For this review, take the finished solid that the model builds, in its own axes (mm). Face numbers are marked on the shaded views. A direction names the side the tool comes from. Round coordinates to 2 decimals unless told otherwise and drop trailing zeros. Loops run counter-clockwise (first coordinate to the right, second up) from the corner with the lowest first, then second, coordinate; pieces in that order, holes last. Notation, with made-up numbers: M -9.5,14 L 31.5,14 A9 ccw 31.5,31 Z; hole C -31,-38.75 d3. An arc over 180 degrees is marked long. Write item = value, one per line. Start each with the question number.
```python
from build123d import *

# Parameters (mm, degrees)
F0_W     = 95.25
F0_H     = 31.75
F1_DEPTH = 88.9
F2_T     = -2.54
F4_D     = 7.9375
F4_DEPTH = 12.7
F5_W     = 15.24
F5_H     = 12.065
F6_DEPTH = 2.54


with BuildPart() as f1:
    # F0 (on Front) → F1 (new body)
    with BuildSketch(Plane.XZ):
        Rectangle(F0_W, F0_H)
    extrude(amount=F1_DEPTH)

    # F2
    f2_openings = [f1.faces().sort_by_distance(p)[0] for p in [
        (0, -44.45, 15.875),
    ]]
    offset(amount=F2_T, openings=f2_openings)

    # F4
    with Locations(Plane.XZ.offset(88.9)):
        with Locations((23.771884, 0)):
            Hole(F4_D / 2, depth=F4_DEPTH)

    # F5 (on face) → F6 (cut, through all)
    with BuildSketch(Plane.XZ.offset(88.9)):
        with Locations((-24.736177, 2.730849)):
            Rectangle(F5_W, F5_H)
    extrude(amount=-F6_DEPTH, mode=Mode.SUBTRACT)


solid = f1.part
```
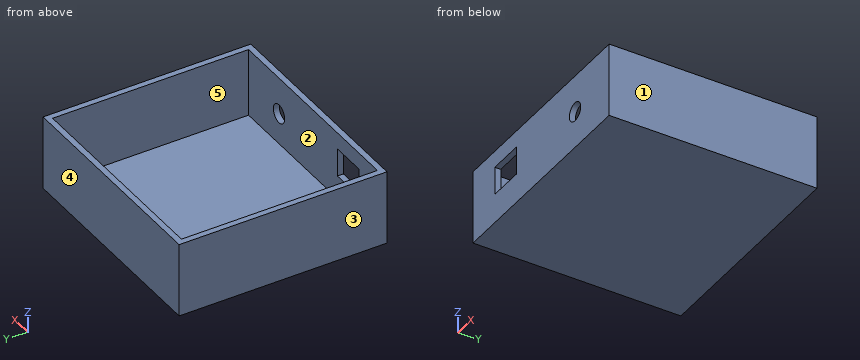
(1) Wall thickness on L1, parallel to Y at x = 10, z = 1; L2, parallel to X at y = -10.5, z = 9 (3 decimals); L3, parallel to Z at x = 19, y = -56 (3 decimals): over which ranges is each line inside the solid? List them lowest first.
(2) For pin 1 Ø5 at (x, z) = (23.77, 0) entering from -Y; pin 2 Ø8 at (x, y) = (-24, -23) entering from +Z (3 decimals), all flat-tipped, find the tip position at first contact; note any pin that passes through.
(3) Add section B-B on x = 21. Write out the cut boundary in (y, z) (3 decimals).
(4) Draft analysis for pull direction X (two halves, no side actions). For the marked faces 3, 4 and 5, state which applies: +X half, -X half, draft (parallel to the pull), parting line (faces both ways), or undercut.
(5) Add section A-A on z = 0. Write out the cut boundary in (x, y) (3 decimals).
(6) Tool access review of the marked faces 1 and 2: name each direction out of +Z, -Z, +X, -X, +Y, -Y from which nothing blocks a thin tool from reaching the whole face with its end or side.
(7) Add section D-D on z = 13.5. Write out the cut boundary in (x, y) (3 decimals), and give its area (3 significant figures).
(8) Add section C-C on x = 35. Write out the cut boundary in (y, z) (3 decimals).
Answer sheet:
q1.L1 = -88.9 to -86.36, -2.54 to 0
q1.L2 = -47.625 to -45.085, 45.085 to 47.625
q1.L3 = -15.875 to -13.335
q2.pin_1 = -2.54
q2.pin_2 = -13.335
q3.outline = M -88.9,-15.875 L 0,-15.875 L 0,15.875 L -2.54,15.875 L -2.54,-13.335 L -86.36,-13.335 L -86.36,-2.84 L -88.9,-2.84 Z; M -88.9,2.84 L -86.36,2.84 L -86.36,15.875 L -88.9,15.875 Z
q4.face_3 = -X half
q4.face_4 = draft
q4.face_5 = undercut
q5.outline = M -47.625,-88.9 L -32.356,-88.9 L -32.356,-86.36 L -45.085,-86.36 L -45.085,-2.54 L 45.085,-2.54 L 45.085,-86.36 L 27.741,-86.36 L 27.741,-88.9 L 47.625,-88.9 L 47.625,0 L -47.625,0 Z; M -17.116,-88.9 L 19.803,-88.9 L 19.803,-86.36 L -17.116,-86.36 Z
q6.face_1 = +Z, -Z, +X, +Y, -Y
q6.face_2 = +Z
q7.outline = M -47.625,-88.9 L 47.625,-88.9 L 47.625,0 L -47.625,0 Z; hole M -45.085,-86.36 L 45.085,-86.36 L 45.085,-2.54 L -45.085,-2.54 Z
q7.area = 910 mm²
q8.outline = M -88.9,-15.875 L 0,-15.875 L 0,15.875 L -2.54,15.875 L -2.54,-13.335 L -86.36,-13.335 L -86.36,15.875 L -88.9,15.875 Z
